Autodesk Inventor part; units mm, degrees
ref_plane "YZ Plane" through (0, 0, 0) normal (1, 0, 0) x (0, 1, 0)
ref_plane "XZ Plane" through (0, 0, 0) normal (0, 1, 0) x (-1, 0, 0)
ref_plane "XY Plane" through (0, 0, 0) normal (0, 0, 1) x (1, 0, 0)
sketch "Sketch1" plane through (0, 0, 0) normal (0, 1, 0) x (-1, 0, 0)
  circle A0 centre (0, 0) radius 8.5
  dimension "d0" = 17
extrude "Extrusion1" add sketch "Sketch1" along normal blind 3
sketch "Sketch2" plane through (0, 3, 0) normal (0, 1, 0) x (1, 0, 0)
  circle A0 centre (0, 0) radius 8.5
  circle A1 centre (0, 0) radius 8
  dimension "d3" = 16
extrude "Extrusion2" add sketch "Sketch2" along normal blind 1.9 contours A1
sketch "Sketch3" plane through (0, 4.9, 0) normal (0, 1, 0) x (1, 0, 0)
  circle A0 centre (0, 0) radius 8
hole "Hole1" at (0, 4.9, 0) direction (0, -1, 0) diameter 12.917 depth 33.1 tip angle 118
properties part number "500-100" material "Steel"
Part model, mm, in its own coordinate system. A direction names the side the tool comes from. Round coordinates to 2 decimals unless told otherwise and drop trailing zeros. Loops run counter-clockwise (first coordinate to the right, second up) from the corner with the lowest first, then second, coordinate; pieces in that order, holes last. Notation, with made-up numbers: (-3, -13.75) -> (7, -13.75) arc R35 ccw to (7, 18.25) -> close; hole circle Ø3 at (54.25, 87). An arc over 180 degrees is marked (long way). Use a Markdown table: item, result.
1) Cut at B-B, the plane z = 0. List the corners of the cut face in (x, y), and give its area (3 significant figures).
The answers:
| item | result |
|---|---|
| outline | (-8.5, 0) -> (-6.46, 0) -> (-6.46, 4.9) -> (-8, 4.9) -> (-8, 3) -> (-8.5, 3) -> close; (6.46, 0) -> (8.5, 0) -> (8.5, 3) -> (8, 3) -> (8, 4.9) -> (6.46, 4.9) -> close |
| area | 18.1 mm2 |
2) Cut at D-D, the plane y = 0.7. List the corners of the cut face in (x, z).
The answers:
| item | result |
|---|---|
| outline | circle Ø17 at (0, 0); hole circle Ø12.92 at (0, 0) |
3) Probe line 1 (Z direction, x = 0, y = 2.6); line 2 (Z direction, x = 0, y = 3.35). List the from-to ranges inside material, lowest first. Write a range as [from, to].
The answers:
| item | result |
|---|---|
| line 1 | z = [-8.5, -6.46], [6.46, 8.5] |
| line 2 | z = [-8, -6.46], [6.46, 8] |
4) Tool access for faces 1 (the cylindrical face through (-1.73, 3.94, -7.81)), 2 (the flat face through (1, 4.9, -7)): list every direction of +Z, -Z, +X, -X, +Y, -Y with a clear straight run to the whole face (end or side of a thin tool).
The answers:
| item | result |
|---|---|
| face 1 | +Y |
| face 2 | +Z, -Z, +X, -X, +Y |
5) Pull direction X, two halves, no side cores. Call faces 3 (the cylindrical face through (-5.446, 2.416, 3.472)), 4 (the flat face through (-6, 0, 3)), 5 (the cylindrical face through (-4.57, 1.479, -7.167)): pulls with the +X half, pulls with the -X half, needs draft (parallel to the pull), parting line crosses it, or undercut.
The answers:
| item | result |
|---|---|
| face 3 | undercut |
| face 4 | needs draft |
| face 5 | parting line crosses it |
6) Cut at A-A, the plane x = 0. List the corners of the cut face in (y, z), and give its area (3 significant figures).
The answers:
| item | result |
|---|---|
| outline | (0, -8.5) -> (3, -8.5) -> (3, -8) -> (4.9, -8) -> (4.9, -6.46) -> (0, -6.46) -> close; (0, 6.46) -> (4.9, 6.46) -> (4.9, 8) -> (3, 8) -> (3, 8.5) -> (0, 8.5) -> close |
| area | 18.1 mm2 |
7) Cut at C-C, the plane y = 3.9. List the corners of the cut face in (x, z), and give its area (3 significant figures).
The answers:
| item | result |
|---|---|
| outline | circle Ø16 at (0, 0); hole circle Ø12.92 at (0, 0) |
| area | 70.0 mm2 |
8) Drop a flat-ended pin along its axis: pin 1 Ø1 at (y, z) = (1.5, -1) entering from +X. Give the stop position or say it passes through.
The answers:
| item | result |
|---|---|
| pin 1 | stops at x = 8.49 |
